Study the drawing (mm; zero at the part's minimum x, y, z) and answer. A direction names the side the tool comes from. Round coordinates to 2 decimals unless told otherwise and drop trailing zeros. Order: outer loops, then holes, each group sorted by start corner. A loop starts at its lowest first (then second) coordinate and runs counter-clockwise, first axis right, second up. Notation, with made-up numbers: (76.5, 18.5) -> (125.5, 18.5) arc R22 ccw to (125.5, 31.5) -> close; hole circle Ø2 at (12, 16). An arc over 180 degrees is marked (long way). Use one line per item in the form item = value.
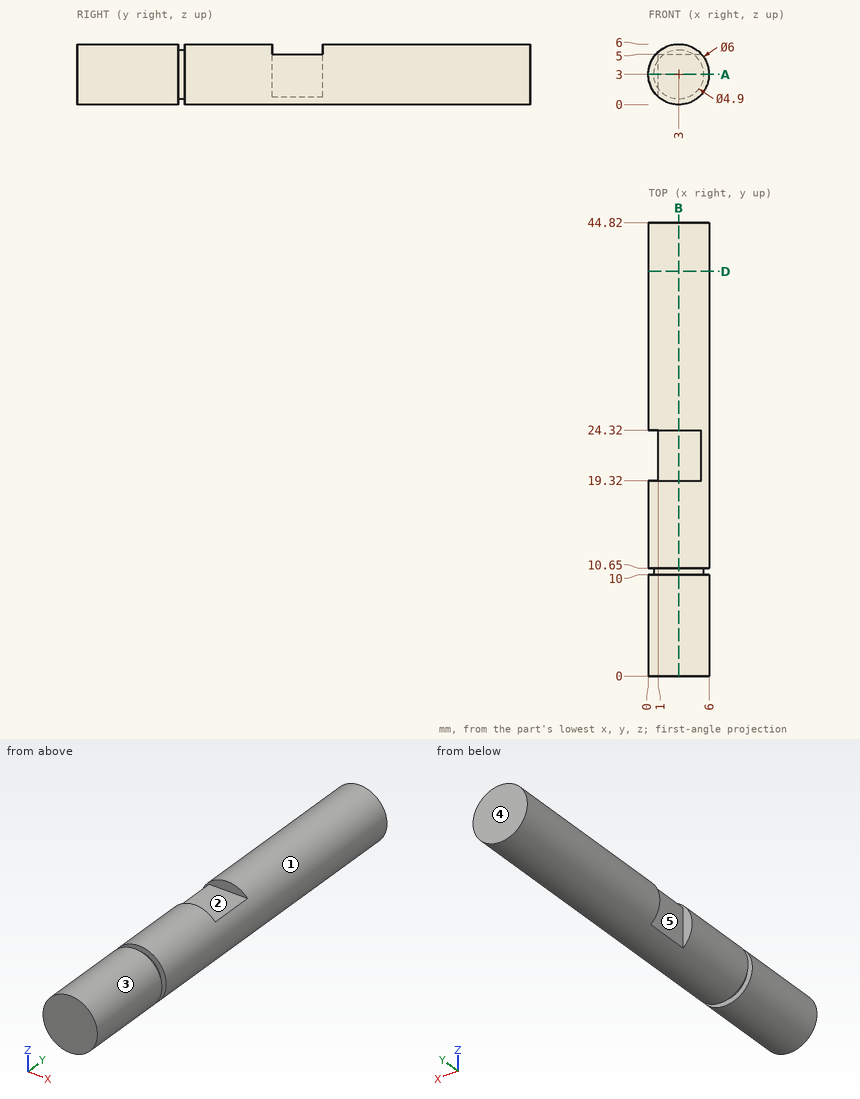
Item 1: Determine the mould class of the marked faces 3, 4 and 5 for opening direction Y: released by +Y, released by -Y, zero draft, split by the parting line, or undercut.
Findings:
face_3 = zero draft
face_4 = released by +Y
face_5 = undercut
Item 2: The part is cut by section D-D, the plane y = 40. Give the vertices of the cut face in (x, z), and give its area (3 significant figures).
Findings:
outline = circle Ø6 at (3, 3)
area = 28.3 mm^2
Item 3: Consider line 1 along Y through (x, z) = (3.5, 0.55); line 2 along Y through (x, z) = (2.75, 5.1); line 3 along Z through (x, y) = (1.7, 39.5). Determine where each line is inside the solid, lowest interval first.
Findings:
line_1 = 0 to 10, 10.65 to 44.82
line_2 = 0 to 19.32, 24.32 to 44.82
line_3 = 0.3 to 5.7
Item 4: Flat-ended cylindrical pins translate along their axes: P1, Ø2, axis at y = 23, z = 3.5, coming from the -X side; P2, Ø1.5, axis at y = 9, z = 5, coming from the +X side; P3, Ø2, axis at x = 2.5, y = 21.5, coming from the +Z side. Find the tip coordinate at first contact, or state that the pin passes through.
Findings:
P1 = 1
P2 = 5.73
P3 = 5
Item 5: The part is cut by section A-A, the plane z = 3. Give the vertices of the cut face in (x, y).
Findings:
outline = (0, 0) -> (6, 0) -> (6, 10) -> (5.45, 10) -> (5.45, 10.65) -> (6, 10.65) -> (6, 44.82) -> (0, 44.82) -> (0, 24.32) -> (1, 24.32) -> (1, 19.32) -> (0, 19.32) -> (0, 10.65) -> (0.55, 10.65) -> (0.55, 10) -> (0, 10) -> close
Item 6: The part is cut by section B-B, the plane x = 3. Give the vertices of the cut face in (y, z), and give its area (3 significant figures).
Findings:
outline = (0, 0) -> (10, 0) -> (10, 0.55) -> (10.65, 0.55) -> (10.65, 0) -> (44.82, 0) -> (44.82, 6) -> (24.32, 6) -> (24.32, 5) -> (19.32, 5) -> (19.32, 6) -> (10.65, 6) -> (10.65, 5.45) -> (10, 5.45) -> (10, 6) -> (0, 6) -> close
area = 263 mm^2
Item 7: For the marked faces 1 and 2, determine the directions among +Z, -Z, +X, -X, +Y, -Y from which every point of the face is accessible in a straight line to the end or side of a thin tool.
Findings:
face_1 = +Y, -Y
face_2 = +Z, +X, -X
